Source: three-view drawing plus pictorial views. Frame: mm from the lowest corner of the part. Coordinates: 2 decimals unless noted, no trailing zeros. Loops run counter-clockwise (first coordinate to the right, second up) from the corner with the lowest first, then second, coordinate; pieces in that order, holes last. Notation, with made-up numbers: M 77.25,78.25 L 120.25,78.25 A24 ccw 120.25,90.25 Z; hole C 66.5,5.5 d4. An arc over 180 degrees is marked long. Use a Markdown table: item, result. Add a question column.
1. Section A-A on x = 29. Output: boundary loops of the cut face in (y, z), then the cut area to 3 significant figures.
2. Section B-B on y = 8. Output: boundary loops of the cut face in (x, z).
3. Pin query (flat end, axial travel): pin 1 (3 mm diameter, centred on x = 50, z = 13.5, fed in from -Y). Return the tip coordinate at first contact, or that it passes through.
4. Line query: L1, parallel to Y at x = 29, z = 12; L2, parallel to X at y = 8, z = 12.5; L3, parallel to Y at x = 28, z = 9.5. Output: solid intervals per line, ascending. Write a range as [from, to].
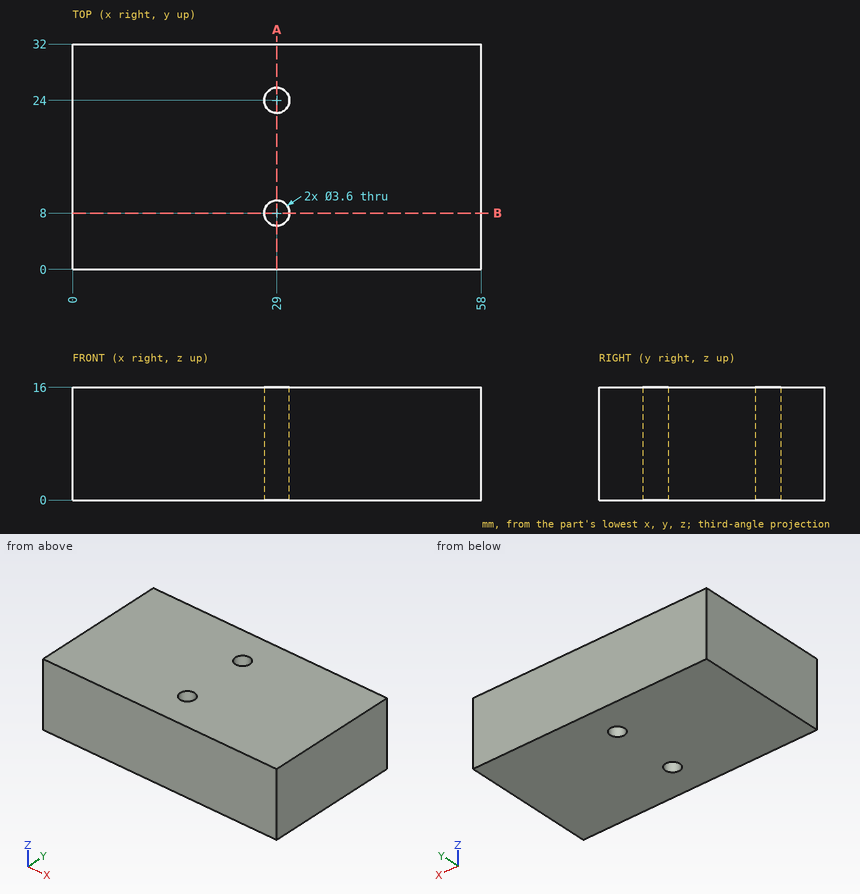
Answers below:
| question | item | result |
|---|---|---|
| 1 | outline | M 0,0 L 6.2,0 L 6.2,16 L 0,16 Z; M 9.8,0 L 22.2,0 L 22.2,16 L 9.8,16 Z; M 25.8,0 L 32,0 L 32,16 L 25.8,16 Z |
| 1 | area | 397 mm² |
| 2 | outline | M 0,0 L 27.2,0 L 27.2,16 L 0,16 Z; M 30.8,0 L 58,0 L 58,16 L 30.8,16 Z |
| 3 | pin 1 | stops at y = 0 |
| 4 | L1 | y = [0, 6.2], [9.8, 22.2], [25.8, 32] |
| 4 | L2 | x = [0, 27.2], [30.8, 58] |
| 4 | L3 | y = [0, 6.5], [9.5, 22.5], [25.5, 32] |
